Source: CAD feature listing. Evaluate the final solid. Frame: model axes, mm. Face numbers are marked on the shaded views. A direction names the side the tool comes from. Coordinates: 2 decimals unless noted, no trailing zeros. Order: outer loops, then holes, each group sorted by start corner. A loop starts at its lowest first (then second) coordinate and runs counter-clockwise, first axis right, second up.
Item 1: Ray query, line 1 (Z direction, x = 0.8, y = -0.85); line 2 (Y direction, x = 0, z = -10.25); line 3 (Z direction, x = 0.45, y = 0.2). Return the intervals inside material, ascending.
Item 2: Reachability of the marked faces 1 and 2 from +Z, -Z, +X, -X, +Y, -Y: full face, straight path, thin tool, end or side. Return the list, or none.
Item 3: Mould query, pull axis Y, two halves, no side actions, for the marked faces 3 and 4. Classes: released by +Y, released by -Y, zero draft, split by the parting line, or undercut.
Item 4: Section A-A on x = 0. Return the cut outline in (y, z).
Item 5: Contact query for a flat-ended pin moving along its axis: P1, Ø1, axis at x = 0.5, z = -11, coming from the +Y side. Output: stop coordinate, or through.
Item 6: Section B-B on z = -4.75. Return the cut outline in (x, y), then the cut area to 3 significant figures.
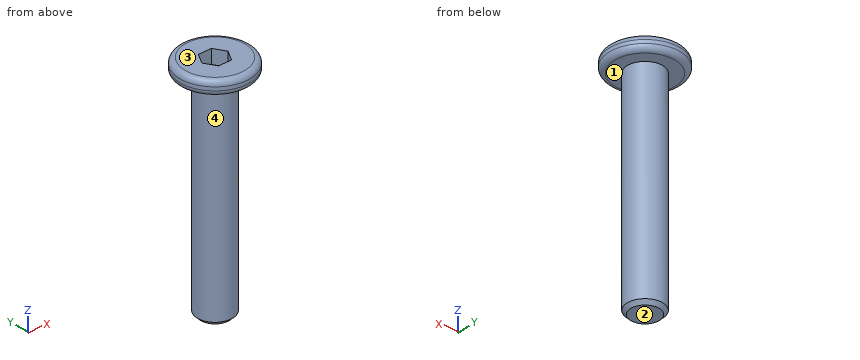
from build123d import *

# Parameters (mm, degrees)
SKETCH_1_R          = 2
EXTRUDE_1_DEPTH     = 0.4
SKETCH_2_R          = 1
EXTRUDE_2_DEPTH     = 12
CHAMFER_1_SIZE      = 0.2
CUT_EXTRUDE_1_DEPTH = 0.8
FILLET_2_R          = 0.3


with BuildPart() as part:
    # 草图1 → 凸台-拉伸1 (new body, symmetric)
    with BuildSketch(Plane.XY):
        Circle(SKETCH_1_R)
    extrude(amount=EXTRUDE_1_DEPTH, both=True)

    # 草图2 → 凸台-拉伸2 (add)
    with BuildSketch(Plane(origin=(0, 0, -0.4), x_dir=(-1, 0, 0), z_dir=(0, 0, -1))):
        Circle(SKETCH_2_R)
    extrude(amount=EXTRUDE_2_DEPTH)

    # 倒角1
    chamfer_1_edges = [part.edges().sort_by_distance(p)[0] for p in [
        (1, 0, -12.4),
    ]]
    chamfer(chamfer_1_edges, length=CHAMFER_1_SIZE)

    # 草图3 → 切除-拉伸1 (cut)
    with BuildSketch(Plane.XY.offset(0.4)):
        Polygon((0.75055535, 0), (0.375277675, 0.65), (-0.375277675, 0.65), (-0.75055535, 0), (-0.375277675, -0.65), (0.375277675, -0.65), align=None)
    extrude(amount=-CUT_EXTRUDE_1_DEPTH, mode=Mode.SUBTRACT)

    # 圆角2
    fillet_2_edges = [part.edges().sort_by_distance(p)[0] for p in [
        (-2, 0, -0.4),
        (-2, 0, 0.4),
    ]]
    fillet(fillet_2_edges, radius=FILLET_2_R)


solid = part.part
Answer list:
1. line 1: z = -0.4 to 0.4
1. line 2: y = -1 to 1
1. line 3: z = -12.4 to -0.4
2. face 1: -Z
2. face 2: -Z, +X, -X, +Y, -Y
3. face 3: zero draft
3. face 4: split by the parting line
4. outline: (-2, -0.1) arc R0.3 ccw to (-1.7, -0.4) - (-1, -0.4) - (-1, -12.2) - (-0.8, -12.4) - (0.8, -12.4) - (1, -12.2) - (1, -0.4) - (1.7, -0.4) arc R0.3 ccw to (2, -0.1) - (2, 0.1) arc R0.3 ccw to (1.7, 0.4) - (0.65, 0.4) - (0.65, -0.4) - (-0.65, -0.4) - (-0.65, 0.4) - (-1.7, 0.4) arc R0.3 ccw to (-2, 0.1) - close
5. P1: stops at y = 1
6. outline: circle Ø2 at (0, 0)
6. area: 3.14 mm2
